Source: CAD feature listing. Evaluate the final solid. Frame: model axes, mm. A direction names the side the tool comes from. Round coordinates to 2 decimals unless told otherwise and drop trailing zeros. Order: outer loops, then holes, each group sorted by start corner. A loop starts at its lowest first (then second) coordinate and runs counter-clockwise, first axis right, second up. Notation, with made-up numbers: M 88.25,53.25 L 112.25,53.25 A21 ccw 112.25,73.25 Z; hole C 12,19.5 d10. An arc over 180 degrees is marked long. Use CSV: the item, a comma, the result in double quotes. Start each with the question number.
```python
from build123d import *

# Parameters (mm, degrees)
EXTRUDE_1_DEPTH             = 50
HOLE_WIZARD_1_D             = 22.1
HOLE_WIZARD_1_DEPTH         = 100
HOLE_WIZARD_2_D             = 3.2
HOLE_WIZARD_2_DEPTH         = 100
HOLE_START                  = -3
HOLE_WIZARD_4_2_4_2_1_DEPTH = 3
RIB_1_REACH                 = 89.542
SKETCH_13_WALL_W            = 200.93798631
SKETCH_13_WALL_H            = 2.1
CHAMFER_1_SIZE              = 3
FILLET_1_R                  = 1.5
FILLET_2_R                  = 1.5


# Read off the part's stored shape, not the designer's step: Ø4.2 (4.2) 直径槽口1
with BuildPart() as part:
    # 草图1 → 凸台-拉伸1 (new body)
    with BuildSketch(Plane.XY):
        Polygon((0, 0), (50.25, 0), (50.25, 48.25), (53.25, 48.25), (53.25, -3), (0, -3), align=None)
    extrude(amount=EXTRUDE_1_DEPTH)

    # 孔1
    with Locations(Plane.ZY.offset(-50.25)):
        with Locations((25, 27.25)):
            Hole(HOLE_WIZARD_1_D / 2, depth=HOLE_WIZARD_1_DEPTH)

    # 孔2
    with Locations(Plane.ZY.offset(-50.25)):
        with Locations((9.5, 42.75), (40.5, 42.75), (40.5, 11.75), (9.5, 11.75)):
            Hole(HOLE_WIZARD_2_D / 2, depth=HOLE_WIZARD_2_DEPTH)

    # Ø4.2 (4.2) 直径槽口1 outline → Ø4.2 (4.2) 直径槽口1 (cut)
    with BuildSketch(Plane(origin=(0, 0, 0), x_dir=(1, 0, 0), z_dir=(0, 1, 0)).offset(HOLE_START)):
        with BuildLine():
            Line((11, -42.1), (41, -42.1))
            ThreePointArc((41, -42.1), (43.1, -40), (41, -37.9))
            Line((41, -37.9), (11, -37.9))
            ThreePointArc((11, -37.9), (8.9, -40), (11, -42.1))
        make_face()
        with BuildLine():
            Line((11, -12.1), (41, -12.1))
            ThreePointArc((41, -12.1), (43.1, -10), (41, -7.9))
            Line((41, -7.9), (11, -7.9))
            ThreePointArc((11, -7.9), (8.9, -10), (11, -12.1))
        make_face()
    extrude(amount=HOLE_WIZARD_4_2_4_2_1_DEPTH, mode=Mode.SUBTRACT)

    # 草图13 wall → 筋1 (add, up to next)
    with BuildSketch(Plane(origin=(43.75, 10, 50), x_dir=(-0.544988350595, -0.838443616301, 0), z_dir=(0.838443616301, -0.544988350595, 0)), mode=Mode.PRIVATE) as rib_1_sk1:
        with Locations((0, 1.05)):
            Rectangle(SKETCH_13_WALL_W, SKETCH_13_WALL_H)
    rib_1_tool1 = extrude(rib_1_sk1.sketch, amount=RIB_1_REACH, mode=Mode.PRIVATE) - part.part
    rib_1 = rib_1_tool1.solids().sort_by_distance((43.75, 10, 50))[0]
    add(rib_1)

    # 镜向1: 筋1 across plane
    add(rib_1.mirror(Plane.XY.offset(25)))

    # 倒角1
    chamfer_1_edges = [part.edges().sort_by_distance(p)[0] for p in [
        (51.75, 48.25, 50),
        (0, -1.5, 50),
        (51.75, 48.25, 0),
        (0, -1.5, 0),
    ]]
    chamfer(chamfer_1_edges, length=CHAMFER_1_SIZE)

    # 圆角1
    fillet_1_edges = [part.edges().sort_by_distance(p)[0] for p in [
        (53.25, -3, 25),
    ]]
    fillet(fillet_1_edges, radius=FILLET_1_R)

    # 圆角2
    fillet_2_edges = [part.edges().sort_by_distance(p)[0] for p in [
        (50.25, 0, 25),
    ]]
    fillet(fillet_2_edges, radius=FILLET_2_R)


solid = part.part
```
(1) Section B-B on z = 25. Return loops of the section in (x, y), plus the area to 3 significant figures.
(2) Section A-A on y = 27.25. Return loops of the section in (x, z).
(3) Contact query for flat-ended pins moving along their axis: P1, Ø14, axis at y = 30.5, z = 23, coming from the -X side; P2, Ø5, axis at y = 42.75, z = 9.5, coming from the -X side. Output: stop coordinate, or through.
(4) Section D-D on y = 11.75. Return loops of the section in (x, z), plus the area to 3 significant figures.
(5) Line query: line 1 along Y through (x, z) = (51, 40); line 2 along Z through (x, y) = (51, 27); line 3 along Z through (x, y) = (51, 42). Output: solid intervals per line, ascending.
(6) Section C-C on z = 9.5. Return loops of the section in (x, y).
(7) Draft query along Y for faces 4 (the face through (49.82, 0.45, 25.32)), 5 (the face through (26, -3, 25)), 6 (the face through (26, -2, 37.9)), 7 (the face through (51.77, 41.19, 9.85)). Return one class per face: pulls with the +Y half, pulls with the -Y half, needs draft (parallel to the pull), parting line crosses it, or undercut.
(8) Reachability of faces 1 (the face through (44, 8, 50)), 2 (the face through (26, -2, 12.1)), 3 (the face through (46, 6, 2.1)) from +Z, -Z, +X, -X, +Y, -Y: full face, straight path, thin tool, end or side. Return the list, or none.
Results below:
1,outline,"M 0,-3 L 51.75,-3 A1.5 ccw 53.25,-1.5 L 53.25,16.2 L 50.25,16.2 L 50.25,1.5 A1.5 cw 48.75,0 L 0,0 Z; M 50.25,38.3 L 53.25,38.3 L 53.25,48.25 L 50.25,48.25 Z"
1,area,"238 mm2"
2,outline,"M 50.25,0 L 53.25,0 L 53.25,13.95 L 50.25,13.95 Z; M 50.25,36.05 L 53.25,36.05 L 53.25,50 L 50.25,50 Z"
3,P1,"passes through"
3,P2,"stops at x = 50.25"
4,outline,"M 44.89,0 L 53.25,0 L 53.25,7.9 L 50.25,7.9 L 50.25,2.1 L 44.89,2.1 Z; M 44.89,47.9 L 50.25,47.9 L 50.25,42.1 L 53.25,42.1 L 53.25,50 L 44.89,50 Z; M 50.25,11.1 L 53.25,11.1 L 53.25,38.9 L 50.25,38.9 Z"
4,area,"153 mm2"
5,line 1,"y = -3 to 10.23, 13.27 to 41.23, 44.27 to 48.25"
5,line 2,"z = 0 to 13.95, 36.05 to 50"
5,line 3,"z = 0 to 8.09, 10.91 to 39.09, 41.91 to 50"
6,outline,"M 0,-3 L 8.96,-3 L 8.96,0 L 0,0 Z; M 43.04,-3 L 51.75,-3 A1.5 ccw 53.25,-1.5 L 53.25,10.15 L 50.25,10.15 L 50.25,1.5 A1.5 cw 48.75,0 L 43.04,0 Z; M 50.25,13.35 L 53.25,13.35 L 53.25,41.15 L 50.25,41.15 Z; M 50.25,44.35 L 53.25,44.35 L 53.25,48.25 L 50.25,48.25 Z"
7,face 4,"pulls with the +Y half"
7,face 5,"pulls with the -Y half"
7,face 6,"needs draft"
7,face 7,"undercut"
8,face 1,"+Z, +X, -X, +Y, -Y"
8,face 2,"+Y, -Y"
8,face 3,"-X, +Y"
